Can you work these out from the model? Positions are in its coordinate system, mm. A direction names the side the tool comes from. Give positions to 0.01 mm unless a question says otherwise; leave off trailing zeros. Write each loop counter-clockwise with the first axis right and the second up, starting at its lowest first coordinate (ties: lowest second). Pieces come first, ordered by that corner, then holes. Notation, with made-up numbers: M 44,-9.75 L 103,-9.75 A19 cw 103,25.25 Z; hole C -19.75,62.25 d5. An arc over 180 degrees is marked long. Write each question's results on one line, items separated by ' | '.
from build123d import *

# Parameters (mm, degrees)
SKETCH1_W           = 300
SKETCH1_H           = 300
BOSS_EXTRUDE1_DEPTH = 300
SKETCH2_W           = 280
SKETCH2_H           = 280
CUT_EXTRUDE1_DEPTH  = 290
SKETCH5_W           = 300
SKETCH5_H           = 300
BOSS_EXTRUDE3_DEPTH = 10
SKETCH6_R           = 100
CUT_EXTRUDE3_DEPTH  = 301
CUT_EXTRUDE4_DEPTH  = 301
CUT_EXTRUDE5_DEPTH  = 10
SKETCH9_R           = 10
BOSS_EXTRUDE4_DEPTH = 35
SKETCH10_R          = 110
SKETCH10_R_2        = 100
BOSS_EXTRUDE5_DEPTH = 30
SKETCH11_R          = 110
SKETCH11_R_2        = 100
BOSS_EXTRUDE6_DEPTH = 30


with BuildPart() as part:
    # Sketch1 → Boss-Extrude1 (new body)
    with BuildSketch(Plane(origin=(0, 0, 0), x_dir=(1, 0, 0), z_dir=(0, 1, 0))):
        Rectangle(SKETCH1_W, SKETCH1_H)
    extrude(amount=BOSS_EXTRUDE1_DEPTH)

    # Sketch2 → Cut-Extrude1 (cut)
    with BuildSketch(Plane(origin=(0, 300, 0), x_dir=(1, 0, 0), z_dir=(0, 1, 0))):
        Rectangle(SKETCH2_W, SKETCH2_H)
    extrude(amount=-CUT_EXTRUDE1_DEPTH, mode=Mode.SUBTRACT)

    # Sketch5 → Boss-Extrude3 (add)
    with BuildSketch(Plane(origin=(0, 300, 0), x_dir=(1, 0, 0), z_dir=(0, 1, 0))):
        Rectangle(SKETCH5_W, SKETCH5_H)
    extrude(amount=-BOSS_EXTRUDE3_DEPTH)

    # Sketch6 → Cut-Extrude3 (cut, through all)
    with BuildSketch(Plane(origin=(0, 300, 0), x_dir=(1, 0, 0), z_dir=(0, 1, 0))):
        Circle(SKETCH6_R)
    extrude(amount=-CUT_EXTRUDE3_DEPTH, mode=Mode.SUBTRACT)

    # Sketch7 → Cut-Extrude4 (cut, through all)
    with BuildSketch(Plane(origin=(0, 0, -150), x_dir=(-1, 0, 0), z_dir=(0, 0, -1))):
        with BuildLine():
            ThreePointArc((100, 150), (70.710678119, 220.710678119), (0, 250))
            Line((0, 250), (0, 50))
            ThreePointArc((0, 50), (70.710678119, 79.289321881), (100, 150))
        make_face()
        with BuildLine():
            Line((0, 50), (0, 250))
            ThreePointArc((0, 250), (-100, 150), (0, 50))
        make_face()
    extrude(amount=-CUT_EXTRUDE4_DEPTH, mode=Mode.SUBTRACT)

    # Sketch8 → Cut-Extrude5 (cut)
    with BuildSketch(Plane.ZY.offset(150)):
        with BuildLine():
            ThreePointArc((0, 250), (-100, 150), (0, 50))
            Line((0, 50), (0, 250))
        make_face()
        with BuildLine():
            Line((0, 250), (0, 50))
            ThreePointArc((0, 50), (70.710678119, 79.289321881), (100, 150))
            ThreePointArc((100, 150), (70.710678119, 220.710678119), (0, 250))
        make_face()
    extrude(amount=-CUT_EXTRUDE5_DEPTH, mode=Mode.SUBTRACT)

    # Sketch9 → Boss-Extrude4 (add)
    with BuildSketch(Plane(origin=(150, 0, 0), x_dir=(0, 0, -1), z_dir=(1, 0, 0))):
        with Locations((140, 290)):
            Circle(SKETCH9_R)
        with Locations((140, 10)):
            Circle(SKETCH9_R)
        with Locations((-140, 290)):
            Circle(SKETCH9_R)
        with BuildLine():
            ThreePointArc((-130, 10), (-132.928932188, 17.071067812), (-140, 20))
            Line((-140, 20), (-140, 0))
            ThreePointArc((-140, 0), (-132.928932188, 2.928932188), (-130, 10))
        make_face()
        with BuildLine():
            Line((-140, 0), (-140, 20))
            ThreePointArc((-140, 20), (-147.071067812, 17.071067812), (-150, 10))
            ThreePointArc((-150, 10), (-147.071067812, 2.928932188), (-140, 0))
        make_face()
    extrude(amount=BOSS_EXTRUDE4_DEPTH)

    # Sketch10 → Boss-Extrude5 (add)
    with BuildSketch(Plane(origin=(0, 300, 0), x_dir=(1, 0, 0), z_dir=(0, 1, 0))):
        Circle(SKETCH10_R)
        Circle(SKETCH10_R_2, mode=Mode.SUBTRACT)
    extrude(amount=BOSS_EXTRUDE5_DEPTH)

    # Sketch11 → Boss-Extrude6 (add)
    with BuildSketch(Plane.XZ):
        Circle(SKETCH11_R)
        Circle(SKETCH11_R_2, mode=Mode.SUBTRACT)
    extrude(amount=BOSS_EXTRUDE6_DEPTH)


solid = part.part
Item 1: If I drill on line 1 (X direction, y = 43.5, z = -133); line 2 (X direction, y = 313.5, z = 0), over which ranges is the centre line in solid material (lowest first)? Write a range as from..to.
Geometry says:
line 1: x = -150..-140, 140..150 | line 2: x = -110..-100, 100..110
Item 2: I want a section at B-B, the plane y = 106. Please give me the cut outline in (x, z), and give its area (3 significant figures).
Geometry says:
outline: M -150,-150 L -89.8,-150 L -89.8,-140 L -140,-140 L -140,-89.8 L -150,-89.8 Z; M -150,89.8 L -140,89.8 L -140,140 L -89.8,140 L -89.8,150 L -150,150 Z; M 89.8,-150 L 150,-150 L 150,150 L 89.8,150 L 89.8,140 L 140,140 L 140,-140 L 89.8,-140 Z | area: 6,210 mm2
Item 3: I'm going to push flat-ended pins straight in: pin 1 (8 mm diameter, centred on y = 164, z = -86.5, fed in from +X); pin 2 (1 mm diameter, centred on x = 139.5, z = 104, fed in from +Y); pin 3 (5 mm diameter, centred on y = 217, z = 30.5, fed in from -X). Where does each tip first touch, or does it pass through?
Geometry says:
pin 1: stops at x = 150 | pin 2: stops at y = 300 | pin 3: stops at x = 140
Item 4: I want a section at A-A, the plane z = 42.5. Please give me the cut outline in (x, y).
Geometry says:
outline: M -150,0 L -101.46,0 L -101.46,-30 L -90.52,-30 L -90.52,10 L -140,10 L -140,59.48 L -150,59.48 Z; M -150,240.52 L -140,240.52 L -140,290 L -90.52,290 L -90.52,330 L -101.46,330 L -101.46,300 L -150,300 Z; M 90.52,-30 L 101.46,-30 L 101.46,0 L 150,0 L 150,300 L 101.46,300 L 101.46,330 L 90.52,330 L 90.52,290 L 140,290 L 140,10 L 90.52,10 Z
Item 5: For faces 1 (the face through (-23.846, 314.79, 107.384)), 2 (the face through (-23.846, -14.79, -107.384)), 3 (the face through (150, 298, 148)), 4 (the face through (-33, 245, 140)), which set-ups out of +Z, -Z, +X, -X, +Y, -Y let a thin tool reach every point of the face, with its end or its side?
Geometry says:
face 1: +Y | face 2: -Y | face 3: +Z, +X, +Y | face 4: none
Item 6: Thinking about a two-plate mould opening in Z: for faces 5 (the face through (65, 300, -102)), 6 (the face through (167.255, 286.17, 130.763)), 7 (the face through (-2, 48, -150)), which applies, +Z half, -Z half, draft (parallel to the pull), parting line (faces both ways), or undercut?
Geometry says:
face 5: draft | face 6: undercut | face 7: -Z half
Item 7: I want a section at D-D, the plane z = -20.5. Please give me the cut outline in (x, y).
Geometry says:
outline: M -150,0 L -108.07,0 L -108.07,-30 L -97.88,-30 L -97.88,10 L -140,10 L -140,52.12 L -150,52.12 Z; M -150,247.88 L -140,247.88 L -140,290 L -97.88,290 L -97.88,330 L -108.07,330 L -108.07,300 L -150,300 Z; M 97.88,-30 L 108.07,-30 L 108.07,0 L 150,0 L 150,300 L 108.07,300 L 108.07,330 L 97.88,330 L 97.88,290 L 140,290 L 140,10 L 97.88,10 Z
Item 8: I want a section at C-C, the plane x = -25. Give the number of separate pieces and of enclosed holes in the cut face, and give its area (3 significant figures).
Geometry says:
separate pieces: 4 | enclosed holes: 0 | area: 5,090 mm2
